Autodesk Inventor part; units mm, degrees
ref_plane "YZ Plane" through (0, 0, 0) normal (1, 0, 0) x (0, 1, 0)
ref_plane "XZ Plane" through (0, 0, 0) normal (0, 1, 0) x (-1, 0, 0)
ref_plane "XY Plane" through (0, 0, 0) normal (0, 0, 1) x (1, 0, 0)
sketch "Sketch1" plane through (0, 0, 0) normal (0, 0, 1) x (1, 0, 0)
  circle A0 centre (0, 0) radius 8
  circle A1 centre (0, 0) radius 4
  dimension "d0" = 16
  dimension "d1" = 8
extrude "Extrusion1" add sketch "Sketch1" along normal blind 7.9
chamfer "Chamfer1" distance 0.7 angle 45 4 edges at (-8, 0, 0) (-8, 0, 7.9) (-4, 0, 0) (-4, 0, 7.9)
sketch "Sketch2" plane through (0, 0, 0) normal (1, 0, 0) x (0, 1, 0)
  line L0 (-4.7, 0) -> (4.7, 0)
  line L1 (4.7, 7.9) -> (-4.7, 7.9)
  point P0 (0, 0)
  point P1 (0, 3.95)
  point P2 (0, 0)
  dimension "d7" = 3.95
hole "Hole1" at (0, 0, 3.95) direction (-1, 0, 0) diameter 2.459 end through all
chamfer "Chamfer2" distance 0.5 angle 45 1 edges at (-8, 0.0002, 5.1795)
properties part number "askraag 8mm" material "Stainless Steel"
Work out the finished part from the listing and answer in its coordinate system (mm). Give positions to 0.01 mm unless a question says otherwise; leave off trailing zeros. Loops run counter-clockwise (first coordinate to the right, second up) from the corner with the lowest first, then second, coordinate; pieces in that order, holes last. Notation, with made-up numbers: (0.25, 31.25) -> (36.25, 31.25) arc R7 ccw to (36.25, 35.25) -> close; hole circle Ø7 at (-37.75, -37.5). An arc over 180 degrees is marked (long way). Put each result on its own line as item: value. Start each with the question number.
Item 1: Find the intervals of material crossed by L1, parallel to X at y = 0, z = 6.25; L2, parallel to X at y = 3, z = 5.75, in increasing order. Write a range as [from, to].
Item 2: The mould has two halves that part along Z. Classify faces 1 (the face through (0, -5, 0)), 2 (the face through (-5.679, -0.369, 2.777)), 3 (the face through (0, -5, 7.9)): released by +Z, released by -Z, zero draft, split by the parting line, or undercut.
Item 3: Each of these flat-tipped pins is pushed along its axis until it touches: P1, Ø6.5, axis at x = 0, y = 0, coming from the +Z side; P2, Ø2, axis at x = 4.5, z = 5.5, coming from the +Y side; P3, Ø3, axis at x = -4.5, z = 1, coming from the +Y side. Where does it stop, or does it pass through?
Item 4: The part is cut by section B-B (y = 0). State how many separate pieces and enclosed holes the cut face has, then the cut area to 3 significant figures.
Item 5: The part is cut by section C-C (z = 6.5). Give the vertices of the cut face in (x, y), then the cut area to 3 significant figures.
Item 6: The part is cut by section A-A (x = 0). Give the vertices of the cut face in (y, z).
Answers below:
1. L1: [-8, -4], [4, 8]
1. L2: [-7.42, -2.65], [2.65, 7.42]
2. face 1: released by -Z
2. face 2: undercut
2. face 3: released by +Z
3. P1: through
3. P2: y = 7.19
3. P3: y = 7.42
4. separate pieces: 3
4. enclosed holes: 0
4. area: 51.2 mm2
5. outline: circle Ø16 at (0, 0); hole circle Ø8 at (0, 0)
5. area: 151 mm2
6. outline: (-8, 0.7) -> (-7.3, 0) -> (-4.7, 0) -> (-4, 0.7) -> (-4, 7.2) -> (-4.7, 7.9) -> (-7.3, 7.9) -> (-8, 7.2) -> close; (4, 0.7) -> (4.7, 0) -> (7.3, 0) -> (8, 0.7) -> (8, 7.2) -> (7.3, 7.9) -> (4.7, 7.9) -> (4, 7.2) -> close
